```python
from build123d import *

# Parameters (mm, degrees)
SZKIC3_R                   = 6
WYTNIJ_WYCI_GNI_CIE1_DEPTH = 30
SFAZOWANIE1_SIZE           = 1.5
SZKIC6_R                   = 2
WYTNIJ_WYCI_GNI_CIE4_DEPTH = 15


with BuildPart() as part:
    # Szkic1 → Obrót1 (revolve)
    with BuildSketch(Plane(origin=(0, 0, 0), x_dir=(1, 0, 0), z_dir=(0, 1, 0))):
        Polygon((-22, 0), (39, 0), (39, 5), (29, 5), (29, 11), (25, 11), (25, 10), (-22, 10), align=None)
    revolve(axis=Axis((-22, 0, 0), (1, 0, 0)))

    # Szkic3 → Wytnij-wyciągnięcie1 (cut)
    with BuildSketch(Plane.ZY.offset(22)):
        Circle(SZKIC3_R)
    extrude(amount=-WYTNIJ_WYCI_GNI_CIE1_DEPTH, mode=Mode.SUBTRACT)

    # Sfazowanie1
    sfazowanie1_edges = [part.edges().sort_by_distance(p)[0] for p in [
        (-22, 0, 10),
    ]]
    chamfer(sfazowanie1_edges, length=SFAZOWANIE1_SIZE)

    # Szkic6 → Wytnij-wyciągnięcie4 (cut, symmetric)
    with BuildSketch(Plane.XY):
        with Locations((35, 0)):
            Circle(SZKIC6_R)
        with Locations((1.5, 0)):
            Circle(SZKIC6_R)
    extrude(amount=WYTNIJ_WYCI_GNI_CIE4_DEPTH, both=True, mode=Mode.SUBTRACT)


solid = part.part
```
Part model, mm, in its own coordinate system. A direction names the side the tool comes from. Coordinates: 2 decimals unless noted, no trailing zeros. Write each loop counter-clockwise with the first axis right and the second up, starting at its lowest first coordinate (ties: lowest second). Pieces come first, ordered by that corner, then holes.
Item 1: Pin check, flat tips, straight feed: pin 1 (5 mm diameter, centred on x = 29, y = 6.5, fed in from +Z); pin 2 (9.5 mm diameter, centred on y = -2, z = 2, fed in from -X); pin 3 (3 mm diameter, centred on x = 13.5, z = -2.5, fed in from -Y); pin 4 (2.5 mm diameter, centred on x = 1.5, y = 0, fed in from -Z). Stop position of each tip, or through.
Item 2: Slice it at A-A (y = 0). Count the separate pieces of the cut face and the enclosed holes in it, and give its area (3 significant figures).
Item 3: Slice it at D-D (x = 35). Write the cut outline in (y, z).
Item 4: Slice it at B-B (z = 0). Write the cut outline in (x, y).
Item 5: Mould opens along X. For faces 4 (the face through (-22, 6, -2)), 5 (the face through (1.24, 1.983, -7.798)), 6 (the face through (26.97, -10.74, 2.38)) say: released by +X, released by -X, zero draft, split by the parting line, or undercut.
Item 6: Which spindle directions (+Z, -Z, +X, -X, +Y, -Y) get a long thin tool onto all of the face, cutting with end or side? Do faces 1 (the face through (1.93, 3, -9.54)), 2 (the face through (39, 0, 0)), 3 (the face through (34, -3, 4)). Say none if no direction does.
Item 7: Slice it at C-C (x = 11). Write the cut outline in (y, z).
Item 8: Probe line 1 (X direction, y = 0, z = 0.75); line 2 (X direction, y = 0, z = -6.7); line 3 (X direction, y = -5.75, z = -8.5). List the from-to ranges inside material, lowest first.
Results found:
1. pin 1: stops at z = 10.25
1. pin 2: stops at x = -22
1. pin 3: stops at y = -9.95
1. pin 4: passes through
2. separate pieces: 4
2. enclosed holes: 0
2. area: 694 mm2
3. outline: (-2, -4.58) - (-2, 4.58) arc R5 ccw to start; (2, -4.58) arc R5 ccw to (2, 4.58) - close
4. outline: (-22, -8.5) - (-20.5, -10) - (25, -10) - (25, -11) - (29, -11) - (29, -5) - (39, -5) - (39, 5) - (29, 5) - (29, 11) - (25, 11) - (25, 10) - (-20.5, 10) - (-22, 8.5) - (-22, 6) - (8, 6) - (8, -6) - (-22, -6) - close; hole circle Ø4 at (35, 0)
5. face 4: released by -X
5. face 5: undercut
5. face 6: zero draft
6. face 1: -X
6. face 2: +Z, -Z, +X, +Y, -Y
6. face 3: +X
7. outline: circle Ø20 at (0, 0)
8. line 1: x = 8 to 33, 37 to 39
8. line 2: x = -22 to -0.5, 3.5 to 29
8. line 3: x = 25 to 29
